```python
from build123d import *

# Parameters (mm, degrees)
ESBO_O1_W                  = 160
ESBO_O1_H                  = 80
RESSALTO_EXTRUS_O1_DEPTH   = 90
ESBO_O2_W                  = 150
ESBO_O2_H                  = 74
CORTE_EXTRUS_O1_DEPTH      = 90
CORTE_EXTRUS_O2_DEPTH      = 90
CORTE_EXTRUS_O3_START      = -3
CORTE_EXTRUS_O3_DEPTH      = 152.536161673
FILETE1_R                  = 10
FILETE2_R                  = 10
RESSALTO_EXTRUS_O3_DEPTH   = 2
ESBO_O14_W                 = 40
ESBO_O14_H                 = 30
RESSALTO_EXTRUS_O10_DEPTH  = 2
FILETE15_R                 = 10
FILETE16_R                 = 10
CORTE_EXTRUS_O8_DEPTH      = 20
CORTE_EXTRUS_O8_DEPTH_BACK = 20
FILETE17_R                 = 10
FILETE18_R                 = 10
FILETE19_R                 = 10
FILETE20_R                 = 10
FILETE21_R                 = 10
FILETE22_R                 = 10
ESBO_O8_W                  = 75
ESBO_O8_H                  = 3
CORTE_EXTRUS_O9_DEPTH      = 77
FILETE24_R                 = 10
FILETE25_R                 = 10
FILETE26_R                 = 10
FILETE27_R                 = 10
ESBO_O9_W                  = 10
ESBO_O9_H                  = 42
RESSALTO_EXTRUS_O11_DEPTH  = 4
ESBO_O17_W                 = 2
ESBO_O17_H                 = 7
ESBO_O17_H_2               = 20
CORTE_EXTRUS_O10_DEPTH     = 10
ESBO_O18_W                 = 10
ESBO_O18_H                 = 42
RESSALTO_EXTRUS_O12_DEPTH  = 4
ESBO_O19_W                 = 2
ESBO_O19_H                 = 7
ESBO_O19_H_2               = 20
CORTE_EXTRUS_O11_DEPTH     = 10


with BuildPart() as part:
    # Esboço1 → Ressalto-extrusão1 (new body)
    with BuildSketch(Plane.XY):
        with Locations((-6.965460526, 3.333333333)):
            Rectangle(ESBO_O1_W, ESBO_O1_H)
    extrude(amount=RESSALTO_EXTRUS_O1_DEPTH)

    # Esboço2 → Corte-extrusão1 (cut)
    with BuildSketch(Plane.XY.offset(90)):
        with Locations((-6.965460526, 3.333333333)):
            Rectangle(ESBO_O2_W, ESBO_O2_H)
    extrude(amount=-CORTE_EXTRUS_O1_DEPTH, mode=Mode.SUBTRACT)

    # Esboço3 → Corte-extrusão2 (cut)
    with BuildSketch(Plane(origin=(0, 43.333333333, 0), x_dir=(1, 0, 0), z_dir=(0, 1, 0))):
        with BuildLine():
            ThreePointArc((-6.965460526, -60), (-49.685479253, -67.746616729), (-86.965460526, -90))
            Line((-86.965460526, -90), (-6.965460526, -90))
            Line((-6.965460526, -90), (-6.965460526, -60))
        make_face()
        with BuildLine():
            Line((-6.965460526, -60), (-6.965460526, -90))
            Line((-6.965460526, -90), (73.034539474, -90))
            ThreePointArc((73.034539474, -90), (35.7545582, -67.746616729), (-6.965460526, -60))
        make_face()
    extrude(amount=-CORTE_EXTRUS_O2_DEPTH, mode=Mode.SUBTRACT)

    # Esboço5 → Corte-extrusão3 (cut, through all)
    with BuildSketch(Plane.XZ.offset(36.666666667).offset(CORTE_EXTRUS_O3_START)):
        with BuildLine():
            ThreePointArc((13.034539474, 61.655093151), (-6.965460526, 60), (-26.965460526, 61.655093151))
            add(Edge.make_bspline(
                [(-26.965460526, 61.655093151), (-6.965460526, -1.655093151), (13.034539474, 61.655093151)],
                knots=[0, 0, 0, 1, 1, 1], degree=2))
        make_face()
    extrude(amount=CORTE_EXTRUS_O3_DEPTH, mode=Mode.SUBTRACT)

    # Filete1
    filete1_edges = [part.edges().sort_by_distance(p)[0] for p in [
        (-26.965460526, -35.166666667, 61.655093151),
    ]]
    fillet(filete1_edges, radius=FILETE1_R)

    # Filete2
    filete2_edges = [part.edges().sort_by_distance(p)[0] for p in [
        (13.034539474, -35.166666667, 61.655093151),
    ]]
    fillet(filete2_edges, radius=FILETE2_R)

    # Esboço7 → Ressalto-extrusão3 (add)
    with BuildSketch(Plane.ZY.offset(5.965460526)):
        Polygon((60, 43.333333333), (0, 43.333333333), (0, -36.666666667), (28, -36.666666667), align=None)
    extrude(amount=RESSALTO_EXTRUS_O3_DEPTH)

    # Esboço14 → Ressalto-extrusão10 (add)
    with BuildSketch(Plane.ZY.offset(5.965460526)):
        with Locations((20, -18.666666667)):
            Rectangle(ESBO_O14_W, ESBO_O14_H)
    extrude(amount=RESSALTO_EXTRUS_O10_DEPTH)

    # Filete15
    # the kernel refuses this fillet: 10 mm, written as the material it adds along each edge
    with BuildSketch(Plane(origin=(-5.965460526, -33.666666667, 0), x_dir=(0, 1, 0), z_dir=(0, 0, 1))) as filete15_piece_1_section:
        with BuildLine():
            CenterArc((FILETE15_R, -FILETE15_R), FILETE15_R, 90, 90)
            Line((0, -FILETE15_R), (0, 0))
            Line((0, 0), (FILETE15_R, 0))
        make_face()
    filete15_piece_1 = extrude(amount=55.079137733, mode=Mode.PRIVATE)
    filete15_piece_1 = split(filete15_piece_1, bisect_by=Plane(origin=(-3.65687296, -31.473045743, 40), z_dir=(0, 0, -1)), keep=Keep.TOP, mode=Mode.PRIVATE)
    add(filete15_piece_1)

    # Filete16
    # the kernel refuses this fillet: 10 mm, written as the material it adds along each edge
    with BuildSketch(Plane(origin=(-7.965460526, -33.666666667, 55.079137733), x_dir=(-1, 0, 0), z_dir=(0, 0, -1))) as filete16_piece_1_section:
        with BuildLine():
            CenterArc((FILETE16_R, FILETE16_R), FILETE16_R, 180, 90)
            Line((0, FILETE16_R), (0, 0))
            Line((0, 0), (FILETE16_R, 0))
        make_face()
    filete16_piece_1 = extrude(amount=55.079137733, mode=Mode.PRIVATE)
    filete16_piece_1 = split(filete16_piece_1, bisect_by=Plane(origin=(-9.937156606, -31.292891496, 40), z_dir=(0, 0, -1)), keep=Keep.TOP, mode=Mode.PRIVATE)
    add(filete16_piece_1)

    # Esboço16 → Corte-extrusão8 (cut, two sides: drawn at the far end of the back side and taken through both)
    with BuildSketch(Plane.ZY.offset(5.965460526).offset(-CORTE_EXTRUS_O8_DEPTH_BACK)):
        Polygon((29, -33.666666667), (58.8, 40.333333333), (60, -33.666666667), align=None)
    extrude(amount=CORTE_EXTRUS_O8_DEPTH + CORTE_EXTRUS_O8_DEPTH_BACK, mode=Mode.SUBTRACT)

    # Filete17
    filete17_edges = [part.edges().sort_by_distance(p)[0] for p in [
        (-81.965460526, 40.333333333, 42.932973789),
    ]]
    fillet(filete17_edges, radius=FILETE17_R)

    # Filete18
    # the kernel refuses this fillet: 10 mm, written as the material it adds along each edge
    with BuildSketch(Plane(origin=(-5.965460526, 40.333333333, 83.8), x_dir=(1, 0, 0), z_dir=(0, 0, -1))) as filete18_piece_1_section:
        with BuildLine():
            CenterArc((FILETE18_R, FILETE18_R), FILETE18_R, 180, 90)
            Line((0, FILETE18_R), (0, 0))
            Line((0, 0), (FILETE18_R, 0))
        make_face()
    filete18_piece_1 = extrude(amount=83.8, mode=Mode.PRIVATE)
    filete18_piece_1 = split(filete18_piece_1, bisect_by=Plane(origin=(-3.682408993, 28.070036468, 53.861537208), z_dir=(0, 0.37355092292184666, -0.927609674369687)), keep=Keep.TOP, mode=Mode.PRIVATE)
    add(filete18_piece_1)

    # Filete19
    filete19_edges = [part.edges().sort_by_distance(p)[0] for p in [
        (68.034539474, 40.333333333, 42.932973789),
    ]]
    fillet(filete19_edges, radius=FILETE19_R)

    # Filete20
    # the kernel refuses this fillet: 10 mm, written as the material it adds along each edge
    with BuildSketch(Plane(origin=(-7.965460526, 40.333333333, 83.8), x_dir=(-1, 0, 0), z_dir=(0, 0, -1))) as filete20_piece_1_section:
        with BuildLine():
            CenterArc((FILETE20_R, -FILETE20_R), FILETE20_R, 90, 90)
            Line((0, -FILETE20_R), (0, 0))
            Line((0, 0), (FILETE20_R, 0))
        make_face()
    filete20_piece_1 = extrude(amount=83.8, mode=Mode.PRIVATE)
    filete20_piece_1 = split(filete20_piece_1, bisect_by=Plane(origin=(-10.248512059, 28.070036468, 53.861537208), z_dir=(0, 0.37355092292187014, -0.9276096743696776)), keep=Keep.TOP, mode=Mode.PRIVATE)
    add(filete20_piece_1)

    # Filete21
    filete21_edges = [part.edges().sort_by_distance(p)[0] for p in [
        (68.034539474, -33.666666667, 42.932973789),
    ]]
    fillet(filete21_edges, radius=FILETE21_R)

    # Filete22
    filete22_edges = [part.edges().sort_by_distance(p)[0] for p in [
        (-81.965460526, -33.666666667, 42.932973789),
    ]]
    fillet(filete22_edges, radius=FILETE22_R)

    # Esboço8 → Corte-extrusão9 (cut)
    with BuildSketch(Plane(origin=(0, 43.333333333, 0), x_dir=(1, 0, 0), z_dir=(0, 1, 0))):
        with Locations((-45.465460526, -35)):
            Rectangle(ESBO_O8_W, ESBO_O8_H)
        with Locations((31.534539474, -35)):
            Rectangle(ESBO_O8_W, ESBO_O8_H)
        with Locations((-45.465460526, -40)):
            Rectangle(ESBO_O8_W, ESBO_O8_H)
        with Locations((31.534539474, -40)):
            Rectangle(ESBO_O8_W, ESBO_O8_H)
    extrude(amount=-CORTE_EXTRUS_O9_DEPTH, mode=Mode.SUBTRACT)

    # Filete24
    filete24_edges = [part.edges().sort_by_distance(p)[0] for p in [
        (73.034539474, -36.666666667, 45),
    ]]
    fillet(filete24_edges, radius=FILETE24_R)

    # Filete25
    filete25_edges = [part.edges().sort_by_distance(p)[0] for p in [
        (-86.965460526, -36.666666667, 45),
    ]]
    fillet(filete25_edges, radius=FILETE25_R)

    # Filete26
    # the kernel refuses this fillet: 10 mm, written as the material it takes off along each edge
    with BuildSketch(Plane(origin=(-86.965460526, 43.333333333, -25), x_dir=(0, -1, 0), z_dir=(0, 0, 1))) as filete26_piece_1:
        with BuildLine():
            CenterArc((FILETE26_R, FILETE26_R), FILETE26_R, 180, 90)
            Line((0, FILETE26_R), (0, 0))
            Line((0, 0), (FILETE26_R, 0))
        make_face()
    extrude(amount=140, mode=Mode.SUBTRACT)

    # Filete27
    # the kernel refuses this fillet: 10 mm, written as the material it takes off along each edge
    with BuildSketch(Plane(origin=(73.034539474, 43.333333333, -25), x_dir=(-1, 0, 0), z_dir=(0, 0, 1))) as filete27_piece_1:
        with BuildLine():
            CenterArc((FILETE27_R, FILETE27_R), FILETE27_R, 180, 90)
            Line((0, FILETE27_R), (0, 0))
            Line((0, 0), (FILETE27_R, 0))
        make_face()
    extrude(amount=140, mode=Mode.SUBTRACT)

    # Esboço9 → Ressalto-extrusão11 (add)
    with BuildSketch(Plane.ZY.offset(86.965460526)):
        with Locations((85, 3.333333333)):
            Rectangle(ESBO_O9_W, ESBO_O9_H)
    extrude(amount=RESSALTO_EXTRUS_O11_DEPTH)

    # Esboço17 → Corte-extrusão10 (cut)
    with BuildSketch(Plane.XY.offset(90)):
        with Locations((-87.965460526, 18.833333333)):
            Rectangle(ESBO_O17_W, ESBO_O17_H)
        with Locations((-87.965460526, 3.333333333)):
            Rectangle(ESBO_O17_W, ESBO_O17_H_2)
        with Locations((-87.965460526, -12.166666667)):
            Rectangle(ESBO_O17_W, ESBO_O17_H)
    extrude(amount=-CORTE_EXTRUS_O10_DEPTH, mode=Mode.SUBTRACT)

    # Esboço18 → Ressalto-extrusão12 (add)
    with BuildSketch(Plane(origin=(73.034539474, 0, 0), x_dir=(0, 0, -1), z_dir=(1, 0, 0))):
        with Locations((-85, 3.333333333)):
            Rectangle(ESBO_O18_W, ESBO_O18_H)
    extrude(amount=RESSALTO_EXTRUS_O12_DEPTH)

    # Esboço19 → Corte-extrusão11 (cut)
    with BuildSketch(Plane.XY.offset(90)):
        with Locations((74.034539474, 18.833333333)):
            Rectangle(ESBO_O19_W, ESBO_O19_H)
        with Locations((74.034539474, 3.333333333)):
            Rectangle(ESBO_O19_W, ESBO_O19_H_2)
        with Locations((74.034539474, -12.166666667)):
            Rectangle(ESBO_O19_W, ESBO_O19_H)
    extrude(amount=-CORTE_EXTRUS_O11_DEPTH, mode=Mode.SUBTRACT)


solid = part.part
```
Input: part model. Units: mm. Frame: model coordinates. A direction names the side the tool comes from. Give positions to 0.01 mm unless a question says otherwise; leave off trailing zeros. Order: outer loops, then holes, each group sorted by start corner. A loop starts at its lowest first (then second) coordinate and runs counter-clockwise, first axis right, second up. Notation, with made-up numbers: M 40.25,28 L 86.25,28 A20 ccw 86.25,52 Z; hole C 81,-34 d1. An arc over 180 degrees is marked long. Return JSON: item names as keys, results as strings.
Item 1: Ray query, probe 1 along X at (y, z) = (12, 25); probe 2 along X at (y, z) = (-7, 40.5); probe 3 along Y at (x, z) = (14.5, 22). Return the intervals inside material, ascending.
Solutions:
{"probe 1": "-86.97 to -81.97, -7.97 to -5.97, 68.03 to 73.03", "probe 2": "-86.97 to -82.97, 69.03 to 73.03", "probe 3": "-36.67 to -33.67, 40.33 to 43.33"}
Item 2: Cut plane D-D (y = -22). Return loops of the section in (x, z), then the cut area to 3 significant figures.
Solutions:
{"outline": "M -86.97,0 L -81.97,0 L -81.97,33.5 L -82.97,33.5 L -82.97,36.5 L -81.97,36.5 L -81.97,38.5 L -82.97,38.5 L -82.97,41.5 L -81.97,41.5 L -81.97,85.87 A121.67 cw -86.97,90 Z; M -7.97,0 L -5.97,0 L -5.97,33.7 L -7.97,33.7 Z; M 68.03,0 L 73.03,0 L 73.03,90 A121.67 cw 68.03,85.87 L 68.03,41.5 L 69.03,41.5 L 69.03,38.5 L 68.03,38.5 L 68.03,36.5 L 69.03,36.5 L 69.03,33.5 L 68.03,33.5 Z", "area": "934 mm^2"}
Item 3: Cut plane B-B (x = 34.5). Return loops of the section in (y, z), then the cut area to 3 significant figures.
Solutions:
{"outline": "M -36.67,0 L -33.67,0 L -33.67,67.28 L -36.67,67.28 Z; M 40.33,0 L 43.33,0 L 43.33,33.5 L 40.33,33.5 Z; M 40.33,36.5 L 43.33,36.5 L 43.33,38.5 L 40.33,38.5 Z; M 40.33,41.5 L 43.33,41.5 L 43.33,67.28 L 40.33,67.28 Z", "area": "386 mm^2"}
Item 4: Cut plane A-A (z = 11). Return loops of the section in (x, y).
Solutions:
{"outline": "M -86.97,-26.67 A10 ccw -76.97,-36.67 L 63.03,-36.67 A10 ccw 73.03,-26.67 L 73.03,33.33 A10 ccw 63.03,43.33 L -76.97,43.33 A10 ccw -86.97,33.33 Z; hole M -81.97,-23.67 A10 ccw -71.97,-33.67 L -17.97,-33.67 A10 ccw -7.97,-23.67 L -7.97,30.33 A10 ccw -17.97,40.33 L -71.97,40.33 A10 ccw -81.97,30.33 Z; hole M -5.97,-23.67 A10 ccw 4.03,-33.67 L 58.03,-33.67 A10 ccw 68.03,-23.67 L 68.03,30.33 A10 ccw 58.03,40.33 L 4.03,40.33 A10 ccw -5.97,30.33 Z"}
Item 5: Pull-direction query (Z, two-part tool) for faces 5 (the flat face through (-7, 6, 0)), 6 (the flat face through (-89, -17.667, 85)), 7 (the flat face through (34, 42, 36.5)); classes: +Z half, -Z half, draft (parallel to the pull), parting line (faces both ways), or undercut.
Solutions:
{"face 5": "-Z half", "face 6": "draft", "face 7": "undercut"}
Item 6: Access query for faces 1 (the flat face through (-8, 43.333, 31)), 2 (the cylindrical face through (-3.11, 37.33, 50.27)), 3 (the flat face through (75, 24.333, 85)), 4 (the flat face through (75.035, -12, 85)). Directions: +Z, -Z, +X, -X, +Y, -Y. A direction counts if a zero-diameter tool reaches every point of the face in a straight line with its end or side. Return the directions, or none.
Solutions:
{"face 1": "+Z, -Z, +X, -X, +Y", "face 2": "+Z, -Z, -Y", "face 3": "+Z, -Z, +X, +Y", "face 4": "+Z, -Z"}
Item 7: Cut plane C-C (y = 28.5). Return loops of the section in (x, z), then the cut area to 3 significant figures.
Solutions:
{"outline": "M -86.97,0 L -81.97,0 L -81.97,33.5 L -82.97,33.5 L -82.97,36.5 L -81.97,36.5 L -81.97,38.5 L -82.97,38.5 L -82.97,41.5 L -81.97,41.5 L -81.97,85.87 A121.67 cw -86.97,90 Z; M -7.97,0 L -5.97,0 L -5.97,54.03 L -7.97,54.03 Z; M 68.03,0 L 73.03,0 L 73.03,90 A121.67 cw 68.03,85.87 L 68.03,41.5 L 69.03,41.5 L 69.03,38.5 L 68.03,38.5 L 68.03,36.5 L 69.03,36.5 L 69.03,33.5 L 68.03,33.5 Z", "area": "975 mm^2"}
Item 8: First-contact query: P1, Ø2.5, axis at y = 22, z = 40.5, coming from the +X side; P2, Ø0.6, axis at x = -88, z = 86, coming from the -Y side; P3, Ø3.5, axis at y = 12, z = 39.5, coming from the -X side. Flat tips, straight axial feed; report the tip coordinate or a pass-through.
Solutions:
{"P1": "x = 73.03", "P2": "y = -17.67", "P3": "x = -86.97"}
